from build123d import *

# Parameters (mm, degrees)
F1_DEPTH = 209.55
F2_W     = 20.6375
F2_H     = 20.6375
F3_DEPTH = 0.4064


# Not quite as in the source:
# - the dataset's text gives a spline's control points without its knots; the knots are read off the source's solid


with BuildPart() as f1:
    # F0 (on Right) → F1 (new body, symmetric)
    with BuildSketch(Plane.YZ):
        Polygon((-139.7, 0), (0, 0), (0, 50.8), (-139.2936, 50.8), (-139.2936, 51.054), (-40.6298144724, 149.7177855276), (-40.9171826682, 150.0051537235), (-139.7, 51.2223363917), align=None)
    extrude(amount=F1_DEPTH, both=True)

    # F2 (on face) → F3 (cut, through all)
    with BuildSketch(Plane(origin=(0, -95.4611681959, 95.4611681959), x_dir=(1, 0, 0), z_dir=(0, -0.7071067812, 0.7071067812))):
        with BuildLine():
            add(Edge.make_bspline(
                [(119.0042372245, 14.038217476), (118.5632678245, 13.597959276), (118.3062706245, 12.977818276), (118.3062706245, 12.354959476)],
                knots=[1, 1, 1, 1, 2, 2, 2, 2], degree=3))
            Line((118.3062706245, 12.354959476), (118.3062706245, 3.623684076))
            add(Edge.make_bspline(
                [(118.3062706245, 3.623684076), (118.3062706245, 3.000114076), (118.5632678245, 2.380023876), (119.0042372245, 1.939740276)],
                knots=[0, 0, 0, 0, 1, 1, 1, 1], degree=3))
            add(Edge.make_bspline(
                [(119.0042372245, 1.939740276), (119.4445462245, 1.498770876), (120.0646618245, 1.242434076), (120.6875206245, 1.242434076)],
                knots=[1, 1, 1, 1, 2, 2, 2, 2], degree=3))
            Line((120.6875206245, 1.242434076), (129.4187706245, 1.242434076))
            add(Edge.make_bspline(
                [(129.4187706245, 1.242434076), (130.0423406245, 1.242434076), (130.6624562245, 1.498770876), (131.1027144245, 1.939740276)],
                knots=[0, 0, 0, 0, 1, 1, 1, 1], degree=3))
            add(Edge.make_bspline(
                [(131.1027144245, 1.939740276), (131.5436838245, 2.380023876), (131.8000206245, 3.000114076), (131.8000206245, 3.623684076)],
                knots=[1, 1, 1, 1, 2, 2, 2, 2], degree=3))
            Line((131.8000206245, 3.623684076), (131.8000206245, 12.354959476))
            add(Edge.make_bspline(
                [(131.8000206245, 12.354959476), (131.8000206245, 12.977818276), (131.5436838245, 13.597959276), (131.1027144245, 14.038217476)],
                knots=[0, 0, 0, 0, 1, 1, 1, 1], degree=3))
            add(Edge.make_bspline(
                [(131.1027144245, 14.038217476), (130.6624562245, 14.479186876), (130.0423406245, 14.736209476), (129.4187706245, 14.736209476)],
                knots=[1, 1, 1, 1, 2, 2, 2, 2], degree=3))
            Line((129.4187706245, 14.736209476), (120.6875206245, 14.736209476))
            add(Edge.make_bspline(
                [(120.6875206245, 14.736209476), (120.0646618245, 14.736209476), (119.4445462245, 14.479186876), (119.0042372245, 14.038217476)],
                knots=[0, 0, 0, 0, 1, 1, 1, 1], degree=3))
        make_face()
        Polygon((-173.3964987755, 56.804959476), (-173.3964987755, 1.242434076), (-103.5464987755, 1.242434076), (-103.5466765755, 56.804959476), align=None)
        Polygon((-91.6402487755, 1.242434076), (-71.0027487755, 1.242434076), (-71.0029265755, 21.879959476), (-91.6404265755, 21.879959476), align=None)
        with Locations((-81.3216765755, 46.486209476)):
            Rectangle(F2_W, F2_H)
        Polygon((32.9785012245, 1.242434076), (102.8281456245, 1.242434076), (102.8281456245, 56.804959476), (32.9781456245, 56.804959476), align=None)
        with BuildLine():
            add(Edge.make_bspline(
                [(-40.5029875755, 15.469304276), (-42.0462153755, 17.012709876), (-44.2145625755, 17.911209476), (-46.3966765755, 17.911209476)],
                knots=[7, 7, 7, 7, 8, 8, 8, 8], degree=3))
            add(Edge.make_bspline(
                [(-46.3966765755, 17.911209476), (-48.5784603755, 17.911209476), (-50.7468075755, 17.012709876), (-52.2898575755, 15.469304276)],
                knots=[0, 0, 0, 0, 1, 1, 1, 1], degree=3))
            add(Edge.make_bspline(
                [(-52.2898575755, 15.469304276), (-53.8329075755, 13.926609876), (-54.7310515755, 11.758262676), (-54.7310515755, 9.576834476), (-54.7310515755, 7.394720476), (-53.8327297755, 5.226373276), (-52.2896797755, 3.682967676)],
                knots=[1, 1, 1, 1, 2, 2, 2, 3, 3, 3, 3], degree=3))
            add(Edge.make_bspline(
                [(-52.2896797755, 3.682967676), (-50.7466297755, 2.140222476), (-48.5782825755, 1.242434076), (-46.3964987755, 1.242434076), (-44.2143847755, 1.242434076), (-42.0460375755, 2.140222476), (-40.5029875755, 3.682967676)],
                knots=[3, 3, 3, 3, 4, 4, 4, 5, 5, 5, 5], degree=3))
            add(Edge.make_bspline(
                [(-40.5029875755, 3.682967676), (-38.9602677755, 5.226373276), (-38.0624793755, 7.394720476), (-38.0624793755, 9.576834476), (-38.0624793755, 11.758262676), (-38.9602677755, 13.926609876), (-40.5029875755, 15.469304276)],
                knots=[5, 5, 5, 5, 6, 6, 6, 7, 7, 7, 7], degree=3))
        make_face()
        with BuildLine():
            add(Edge.make_bspline(
                [(169.6082508245, 16.824597476), (167.9183888245, 18.514789676), (165.5433618245, 19.498709476), (163.1535012245, 19.498709476)],
                knots=[7, 7, 7, 7, 8, 8, 8, 8], degree=3))
            add(Edge.make_bspline(
                [(163.1535012245, 19.498709476), (160.7636406245, 19.498709476), (158.3889184245, 18.514789676), (156.6991072245, 16.824597476)],
                knots=[0, 0, 0, 0, 1, 1, 1, 1], degree=3))
            add(Edge.make_bspline(
                [(156.6991072245, 16.824597476), (155.0092706245, 15.135141876), (154.0253762245, 12.760114876), (154.0253762245, 10.370584476), (154.0253762245, 7.980368276), (155.0092706245, 5.605315876), (156.6991072245, 3.915834876)],
                knots=[1, 1, 1, 1, 2, 2, 2, 3, 3, 3, 3], degree=3))
            add(Edge.make_bspline(
                [(156.6991072245, 3.915834876), (158.3889184245, 2.225668076), (160.7636406245, 1.242434076), (163.1535012245, 1.242434076), (165.5433618245, 1.242434076), (167.9183888245, 2.225668076), (169.6082508245, 3.915834876)],
                knots=[3, 3, 3, 3, 4, 4, 4, 5, 5, 5, 5], degree=3))
            add(Edge.make_bspline(
                [(169.6082508245, 3.915834876), (171.2980366245, 5.605315876), (172.2816262245, 7.980368276), (172.2816262245, 10.370584476), (172.2816262245, 12.760114876), (171.2980366245, 15.135141876), (169.6082508245, 16.824597476)],
                knots=[5, 5, 5, 5, 6, 6, 6, 7, 7, 7, 7], degree=3))
        make_face()
    extrude(amount=-F3_DEPTH, mode=Mode.SUBTRACT)


solid = f1.part
Could you check a few things on this model? Use its own coordinates, in mm. A direction names the side the tool comes from. Round coordinates to 2 decimals unless told otherwise and drop trailing zeros. Write each loop counter-clockwise with the first axis right and the second up, starting at its lowest first coordinate (ties: lowest second). Pieces come first, ordered by that corner, then holes. Notation, with made-up numbers: (-37, 4) - (-23, 4) arc R23 ccw to (-23, 28) - close; hole circle Ø11 at (66.5, -24). An arc over 180 degrees is marked (long way). Put each result on its own line as item: value. Start each with the question number.
(1) For faces 1 (the flat face through (-173.396, -74.5, 116.1)), 2 (the flat face through (3, -69, 50.8)), 3 (the flat face through (3, 0, 25)), which set-ups out of +Z, -Z, +X, -X, +Y, -Y let a thin tool reach every point of the face, with its end or its side?
(2) Thinking about a two-plate mould opening in Z: for faces 4 (the flat face through (2.934, -89.617, 101.305)), 5 (the flat face through (2.93, -90.65, 99.7)), 6 (the flat face through (3, -139.7, 26)), which applies, released by +Z, released by -Z, zero draft, split by the parting line, or undercut?
(3) I want a section at B-B, the plane x = -169.5. Please give me the cut outline in (y, z), plus the area to 3 significant figures.
(4) I want a section at C-C, the plane y = -124. Please give me the cut outline in (x, z), plus the area to 3 significant figures.
(5) I need wall thicknesses on probe 1 along Z at (x, y) = (-122, -34.5); probe 2 along Z at (x, y) = (41.5, -124.5); probe 3 along Z at (x, y) = (-81, -119). Which ranges of each line are inside material? Lowest first, please.
(6) I want a section at D-D, the plane x = 138. Please give me the cut outline in (y, z), plus the area to 3 significant figures.
(7) I want a section at A-A, the plane x = -86. Please give me the cut outline in (y, z), plus the area to 3 significant figures.
(8) Will these pins go through, and if not, where does the flat tip stop? pin 1 (1.9 mm diameter, centred on y = -90, z = 101.5, fed in from -X); pin 2 (8 mm diameter, centred on x = -75, y = -78.5, fed in from +Z); pin 3 (10 mm diameter, centred on x = 34, y = -114, fed in from +Z); pin 4 (3 mm diameter, centred on x = 78.5, y = -23.5, fed in from +Z).
Here are the results:
1. face 1: +Z, +Y, -Y
1. face 2: +X, -X, +Y
1. face 3: +Z, -Z, +X, -X, +Y
2. face 4: released by +Z
2. face 5: undercut
2. face 6: zero draft
3. outline: (-139.7, 0) - (0, 0) - (0, 50.8) - (-139.29, 50.8) - (-139.29, 51.05) - (-94.3, 96.05) - (-94.58, 96.34) - (-139.7, 51.22) - close; (-55.29, 135.63) - (-55.01, 135.34) - (-40.63, 149.72) - (-40.92, 150.01) - close
3. area: 7,130 mm^2
4. outline: (-209.55, 0) - (209.55, 0) - (209.55, 50.8) - (-209.55, 50.8) - close; (-209.55, 66.35) - (209.55, 66.35) - (209.55, 66.92) - (-209.55, 66.92) - close
4. area: 21,500 mm^2
5. probe 1: z = 0 to 50.8
5. probe 2: z = 0 to 50.8, 65.85 to 66.42
5. probe 3: z = 0 to 50.8, 71.35 to 71.92
6. outline: (-139.7, 0) - (0, 0) - (0, 50.8) - (-139.29, 50.8) - (-139.29, 51.05) - (-40.63, 149.72) - (-40.92, 150.01) - (-139.7, 51.22) - close
6. area: 7,150 mm^2
7. outline: (-139.7, 0) - (0, 0) - (0, 50.8) - (-139.29, 50.8) - (-139.29, 51.05) - (-94.3, 96.05) - (-94.58, 96.34) - (-139.7, 51.22) - close; (-79.99, 110.93) - (-79.7, 110.65) - (-69.6, 120.75) - (-69.89, 121.04) - close; (-55.29, 135.63) - (-55.01, 135.34) - (-40.63, 149.72) - (-40.92, 150.01) - close
7. area: 7,140 mm^2
8. pin 1: stops at x = -209.55
8. pin 2: stops at z = 116.42
8. pin 3: stops at z = 81.92
8. pin 4: stops at z = 50.8
